Check sheet for the modelled part. Datum: model origin and axes. Units: mm. A direction names the side the tool comes from. Round coordinates to 2 decimals unless told otherwise and drop trailing zeros. Write each loop counter-clockwise with the first axis right and the second up, starting at its lowest first coordinate (ties: lowest second). Pieces come first, ordered by that corner, then holes.
Item 1: Release check for a two-part mould opening along X. For faces 6 (the flat face through (-80, 16, 0)), 7 (the flat face through (82.05, 4, 8)), 8 (the flat face through (79, 23, 15)) record: +X half, -X half, draft (parallel to the pull), parting line (faces both ways), or undercut.
Item 2: Cross-section at C-C on y = 25. Enter the section's corners in (x, z).
Item 3: Cross-section at A-A on x = 0. Enter the section's corners in (y, z), plus the area to 3 significant figures.
Item 4: Material ranges on line 1 (X direction, y = 10.5, z = 12); line 2 (Z direction, x = 0, y = 38); line 3 (X direction, y = 29, z = -12.75), recorded low to high.
Item 5: Cross-section at B-B on z = 0. Enter the section's corners in (x, y), plus the area to 3 significant figures.
Item 6: Cross-section at D-D on x = 57.5. Enter the section's corners in (y, z).
Item 7: Tool access check on faces 1 (the conical face through (-1.123, 43.93, 8.554)), 2 (the flat face through (84.65, 4, 8)), 3 (the cylindrical face through (-80.86, 3.94, 4.58)), 4 (the flat face through (-78.5, 16, 0)), 5 (the cylindrical face through (87.932, 7.892, 11.456)). Record the directions out of +Z, -Z, +X, -X, +Y, -Y that give a thin tool (end or side, any length) a straight path to the whole face; none if there is none.
Item 8: Go/stop test with flat-tipped pins: pin 1 Ø1.6 at (x, y) = (47, 34) entering from +Z; pin 2 Ø2 at (x, z) = (33.5, -3.5) entering from -Y; pin 3 Ø12 at (x, y) = (75, 8) entering from +Z; pin 4 Ø1.2 at (y, z) = (34, -7.5) entering from -X. Record where each tip stops, or that it passes through.
Autodesk Inventor part; units mm, degrees
ref_plane "Plan de construction4" through (-84.65, 8, 9) normal (-1, 0, 0) x (0, 0, 1)
ref_plane "Plan de construction5" through (-78, 34.25, 15) normal (0, 1, 0) x (1, 0, 0)
ref_plane "Plan de construction6" through (86.65, 8, 9) normal (1, 0, 0) x (0, 0, -1)
sketch "Esquisse1" plane through (0, 0, 0) normal (0, 0, 1) x (1, 0, 0)
  line L0 (-80, 0) -> (-80, 35)
  line L1 (-80, 35) -> (80, 35)
  line L2 (80, 35) -> (80, 0)
  line L3 (80, 0) -> (78.5, 0)
  line L4 (78.5, 0) -> (78.5, 33.5)
  line L5 (78.5, 33.5) -> (-78.5, 33.5)
  line L6 (-78.5, 33.5) -> (-78.5, 0)
  line L7 (-78.5, 0) -> (-80, 0)
  point P0 (0, 0)
  point P1 (-79.25, 0)
  point P2 (0, 35)
  point P3 (0, 33.5)
  dimension "d0" = 1.5
  dimension "d1" = 1.5
  dimension "d2" = 160
  dimension "d3" = 35
extrude "Extrusion1" add sketch "Esquisse1" along normal mid plane 30
fillet "Congé1" radius 2 2 edges at (80, 35, 0) (-80, 35, 0)
fillet "Congé1" radius 1 2 edges at (-78.5, 33.5, 0) (78.5, 33.5, 0)
sketch "Esquisse2" plane through (-78, 35, 15) normal (0, 1, 0) x (1, 0, 0)
  line L0 (64.3632, 4.6) -> (91.6368, 4.6)
  line L1 (91.6368, 25.4) -> (64.3632, 25.4)
  arc A0 (64.3632, 25.4) -> (64.3632, 4.6) centre (78, 15) ccw
  arc A1 (91.6368, 4.6) -> (91.6368, 25.4) centre (78, 15) ccw
  point P0 (102.0926, 15)
  dimension "d9" = 20.8
  dimension "d10" = 17.15
  dimension "d11" = 17.15
  dimension "d12" = 10.4
extrude "Extrusion2" add sketch "Esquisse2" along normal blind 4
sketch "Esquisse3" plane through (-78, 39, 15) normal (0, 1, 0) x (1, 0, 0)
  circle A0 centre (78, 15) radius 8.75
  dimension "d15" = 17.5
extrude "Extrusion3" add sketch "Esquisse3" along normal blind 10 draft -1.43
sketch "Esquisse6" plane through (-80, 0, -15) normal (-1, 0, 0) x (0, 0, 1)
  circle A0 centre (24, 8) radius 6
  line L0 (30, 33) -> (30, 0)
  point P0 (15, 0)
  dimension "d20" = 12
  dimension "d21" = 8
extrude "Extrusion4" add sketch "Esquisse6" along normal blind 6.65
ref_plane "Plan de construction4" through (-84.65, 8, 9) normal (-1, 0, 0) x (0, 0, 1)
sketch "Esquisse7" plane through (-84.65, 8, 9) normal (-1, 0, 0) x (0, 0, 1)
  circle A0 centre (0, 0) radius 6 construction
  circle A1 centre (0, 0) radius 3.75
  circle A2 centre (0, 0) radius 7
  point P0 (-9, -8)
  point P1 (6, 0)
  dimension "d25" = 7.5
  dimension "d26" = 1
extrude "Extrusion5" cut sketch "Esquisse7" against normal blind 2.6
mirror "Symétrie2" about plane through (0, 0, 0) normal (1, 0, 0) of "Extrusion4", "Extrusion5"
sketch "Esquisse8" plane through (-78, 35, 15) normal (0, 1, 0) x (1, 0, 0)
  line L0 (18.2, 21.5) -> (43, 21.5)
  line L1 (43, 21.5) -> (43, 30)
  line L2 (43, 30) -> (18.2, 30)
  line L3 (18.2, 30) -> (18.2, 21.5)
  line L4 (113, 21.5) -> (137.8, 21.5)
  line L5 (137.8, 21.5) -> (137.8, 30)
  line L6 (137.8, 30) -> (113, 30)
  line L7 (113, 30) -> (113, 21.5)
  line L8 (113, 0) -> (137.8, 0)
  line L9 (137.8, 0) -> (137.8, 8.5)
  line L10 (137.8, 8.5) -> (113, 8.5)
  line L11 (113, 8.5) -> (113, 0)
  line L12 (18.2, 0) -> (43, 0)
  line L13 (43, 0) -> (43, 8.5)
  line L14 (43, 8.5) -> (18.2, 8.5)
  line L15 (18.2, 8.5) -> (18.2, 0)
  line L16 (0, 30) -> (156, 30)
  line L17 (156, 0) -> (0, 0)
  point P0 (78, 15)
  dimension "d32" = 24.8
  dimension "d33" = 24.8
  dimension "d34" = 70
  dimension "d35" = 35
  dimension "d36" = 8.5
  dimension "d37" = 8.5
extrude "Extrusion6" cut sketch "Esquisse8" against normal through all
sketch "Esquisse9" plane through (78, 35, 15) normal (0, 1, 0) x (1, 0, 0)
  line L0 (-137.8, 23.9) -> (-113, 23.9)
  line L1 (-113, 23.9) -> (-113, 26.4)
  line L2 (-113, 26.4) -> (-137.8, 26.4)
  line L3 (-137.8, 26.4) -> (-137.8, 23.9)
  line L4 (-137.8, 3.6) -> (-113, 3.6)
  line L5 (-113, 3.6) -> (-113, 6.1)
  line L6 (-113, 6.1) -> (-137.8, 6.1)
  line L7 (-137.8, 6.1) -> (-137.8, 3.6)
  line L8 (-43, 23.9) -> (-18.2, 23.9)
  line L9 (-18.2, 23.9) -> (-18.2, 26.4)
  line L10 (-18.2, 26.4) -> (-43, 26.4)
  line L11 (-43, 26.4) -> (-43, 23.9)
  line L12 (-43, 3.6) -> (-18.2, 3.6)
  line L13 (-18.2, 3.6) -> (-18.2, 6.1)
  line L14 (-18.2, 6.1) -> (-43, 6.1)
  line L15 (-43, 6.1) -> (-43, 3.6)
  line L16 (-137.8, 21.5) -> (-137.8, 30)
  line L17 (-113, 30) -> (-113, 21.5)
  line L18 (-43, 21.5) -> (-43, 30)
  line L19 (-18.2, 30) -> (-18.2, 21.5)
  line L20 (-113, 21.5) -> (-137.8, 21.5)
  line L21 (-137.8, 8.5) -> (-113, 8.5)
  point P0 (-78, 15)
  dimension "d40" = 2.5
  dimension "d41" = 2.5
  dimension "d42" = 2.4
  dimension "d43" = 2.4
extrude "Extrusion7" add sketch "Esquisse9" against normal up to surface (1.5 mm away) contours L3 L2 L1 L0 | L7 L6 L5 L4 | L11 L10 L9 L8 | L15 L14 L13 L12
sketch "Esquisse10" plane through (0, 49, 0) normal (0, 1, 0) x (1, 0, 0)
  point P0 (0, 0)
  point P1 (0, 0)
hole "Perçage1" at (0, 49, 0) direction (0, -1, 0) diameter 8 end through all
ref_plane "Plan de construction5" through (-78, 34.25, 15) normal (0, 1, 0) x (1, 0, 0)
sketch "Esquisse11" plane through (-78, 34.25, 15) normal (0, 1, 0) x (1, 0, 0)
  line L0 (18.2, 23.9) -> (43, 23.9) construction
  line L1 (43, 26.4) -> (18.2, 26.4) construction
  line L2 (18.2, 3.6) -> (43, 3.6) construction
  line L3 (43, 6.1) -> (18.2, 6.1) construction
  line L4 (-59.7354, 25.15) -> (184.2548, 25.15)
  line L5 (-24.0556, 4.85) -> (192.1599, 4.85)
  point P0 (78, 15)
  dimension "d53" = 2.5
  dimension "d54" = 2.5
  dimension "d55" = 1.25
  dimension "d56" = 1.25
ref_plane "Plan de construction6" through (86.65, 8, 9) normal (1, 0, 0) x (0, 0, -1)
sketch "Esquisse13" plane through (86.65, 8, 9) normal (1, 0, 0) x (0, 0, -1)
  circle A0 centre (0, 0) radius 6
  circle A1 centre (0, 0) radius 6 construction
  point P0 (9, -8)
extrude "Extrusion8" add sketch "Esquisse13" along normal blind 6.5
sketch "Esquisse14" plane through (93.15, 8, 9) normal (1, 0, 0) x (0, 0, -1)
  circle A0 centre (0, 0) radius 6 construction
  point P0 (9, -8)
hole "Perçage2" at (93.15, 8, 9) direction (-1, 0, 0) diameter 4.917 depth 10 tip angle 118
chamfer "Chanfrein2" distance 0.3 angle 45 7 edges at (93.15, 8, 15) (93.15, 8, 11.4585) (84.65, 8, 3) (82.05, 8, 3) (-84.65, 8, 3) (-86.65, 8, 3) (-82.05, 8, 3)
equation "\"d1\" = d0"
equation "\"d11\" = d10"
equation "\"d33\" = d32"
equation "\"d37\" = d36"
equation "\"d41\" = d40"
equation "\"d43\" = d42"
equation "\"d55\" = 0.5 * d53"
equation "\"d56\" = 0.5 * d54"
equation "\"nombredor\" = 1.61803"
equation "\"pi\" = 3.141593"
properties part number "Maintient courvercle" material "Acier inoxydable"
Response values:
1. face 6: -X half
1. face 7: undercut
1. face 8: draft
2. outline: (-80, -15) - (-78.5, -15) - (-78.5, 15) - (-80, 15) - close; (78.5, -15) - (80, -15) - (80, 15) - (78.5, 15) - close
3. outline: (33.5, -15) - (35, -15) - (35, -10.4) - (39, -10.4) - (39, -8.75) - (49, -8.5) - (49, -4) - (33.5, -4) - close; (33.5, 4) - (49, 4) - (49, 8.5) - (39, 8.75) - (39, 10.4) - (35, 10.4) - (35, 15) - (33.5, 15) - close
3. area: 177 mm2
4. line 1: x = -86.65 to -84.65, -82.05 to -78.5, 78.5 to 82.05, 84.65 to 93.15
4. line 2: z = -10.4 to -4, 4 to 10.4
4. line 3: x = -80 to -78.5, 78.5 to 80
5. outline: (-80, 0) - (-78.5, 0) - (-78.5, 32.5) arc R1 cw to (-77.5, 33.5) - (-4, 33.5) - (-4, 49) - (-8.5, 49) - (-8.75, 39) - (-17.15, 39) - (-17.15, 35) - (-78, 35) arc R2 ccw to (-80, 33) - close; (4, 33.5) - (77.5, 33.5) arc R1 cw to (78.5, 32.5) - (78.5, 0) - (80, 0) - (80, 33) arc R2 ccw to (78, 35) - (17.15, 35) - (17.15, 39) - (8.75, 39) - (8.5, 49) - (4, 49) - close
5. area: 525 mm2
6. outline: (33.5, -11.4) - (35, -11.4) - (35, -8.9) - (33.5, -8.9) - close; (33.5, -6.5) - (35, -6.5) - (35, 6.5) - (33.5, 6.5) - close; (33.5, 8.9) - (35, 8.9) - (35, 11.4) - (33.5, 11.4) - close
7. face 1: +Y
7. face 2: none
7. face 3: -X
7. face 4: +Z, -Z, -Y
7. face 5: +X
8. pin 1: stops at z = 11.4
8. pin 2: stops at y = 33.5
8. pin 3: stops at z = 15
8. pin 4: stops at x = -79.96
